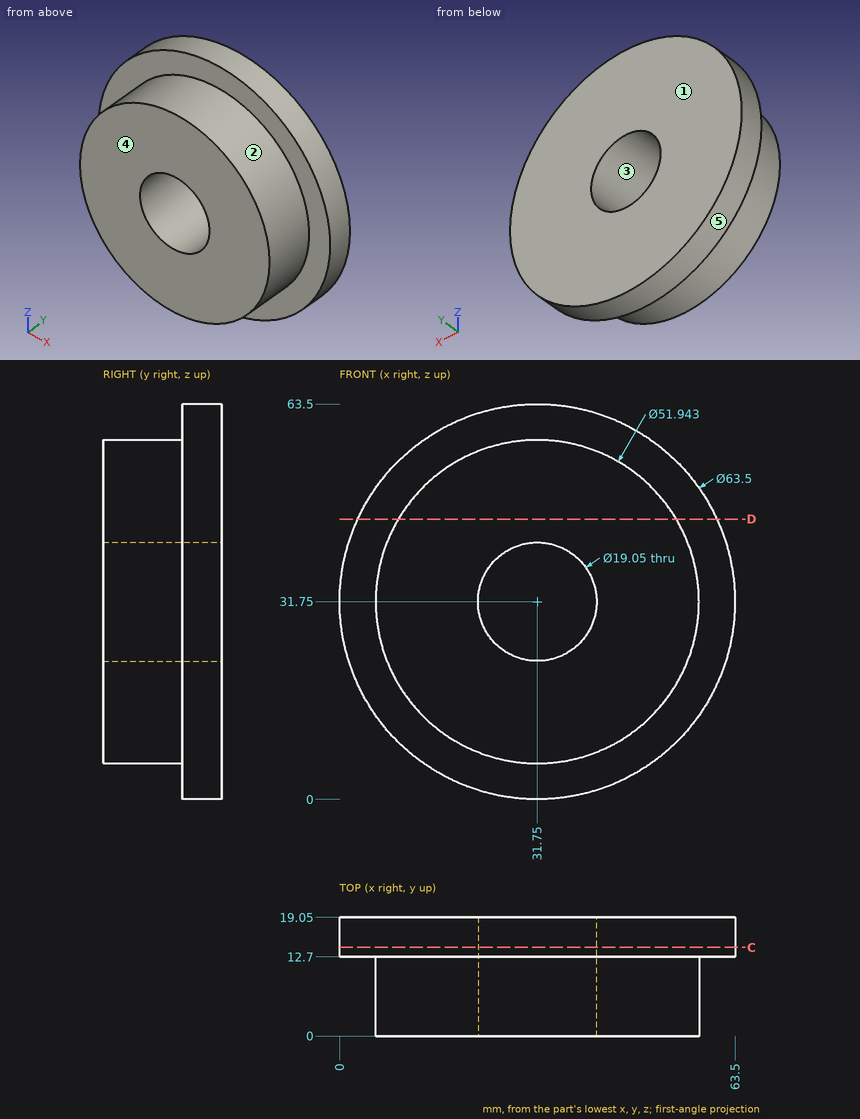
The figure shows three views and two pictorial views of one solid part (mm, origin at its lowest corner). Answer the questions. A direction names the side the tool comes from. Round coordinates to 2 decimals unless told otherwise and drop trailing zeros. Write each loop counter-clockwise with the first axis right and the second up, starting at its lowest first coordinate (ties: lowest second). Pieces come first, ordered by that corner, then holes. Notation, with made-up numbers: M 54,32.25 L 81,32.25 A28 cw 81,58.25 Z; hole C 72.25,54 d1. An arc over 180 degrees is marked long. Use a Markdown table: item, result.
1) Flat-ended cylindrical pins translate along their axes: pin 1 (1.5 mm diameter, centred on x = 18.5, y = 7.5, fed in from +Z); pin 2 (2 mm diameter, centred on x = 48, y = 4.5, fed in from +Z); pin 3 (1 mm diameter, centred on x = 48, y = 2, fed in from +Z). Find the tip coordinate at first contact, or state that the pin passes through.
Answers follow:
| item | result |
|---|---|
| pin 1 | stops at z = 54.52 |
| pin 2 | stops at z = 52.77 |
| pin 3 | stops at z = 52.4 |
2) The part is cut by section D-D (z = 45). Write down the section's boundary in (x, y).
Answers follow:
| item | result |
|---|---|
| outline | M 2.9,12.7 L 9.41,12.7 L 9.41,0 L 54.09,0 L 54.09,12.7 L 60.6,12.7 L 60.6,19.05 L 2.9,19.05 Z |
3) The part is cut by section C-C (y = 14.25). Write down the section's boundary in (x, z) (3 decimals), plus the area to 3 significant figures.
Answers follow:
| item | result |
|---|---|
| outline | C 31.75,31.75 d63.5; hole C 31.75,31.75 d19.05 |
| area | 2,880 mm2 |
4) For a pull along X with two mould halves and no side action, classify the marked faces 3, 4 and 5 as pulls with the +X half, pulls with the -X half, needs draft (parallel to the pull), parting line crosses it, or undercut.
Answers follow:
| item | result |
|---|---|
| face 3 | undercut |
| face 4 | needs draft |
| face 5 | parting line crosses it |
5) A tool of negligible diameter and unlimited length cuts with its end or side. For the marked faces 1 and 2, from which of +Z, -Z, +X, -X, +Y, -Y can it reach the whole face along a straight path? Write none if from no direction.
Answers follow:
| item | result |
|---|---|
| face 1 | +Z, -Z, +X, -X, +Y |
| face 2 | -Y |
6) Straight lines are drawn through the part: line 1 along Z through (x, y) = (31.75, 13.25) (3 decimals); line 2 along Z through (x, y) = (31.75, 12) (1 decimal); line 3 along X through (y, z) = (9.25, 28.5). For each, find the intervals that lie inside material, in ascending order. Write a range as [from, to].
Answers follow:
| item | result |
|---|---|
| line 1 | z = [0, 22.225], [41.275, 63.5] |
| line 2 | z = [5.8, 22.2], [41.3, 57.7] |
| line 3 | x = [5.98, 22.8], [40.7, 57.52] |
